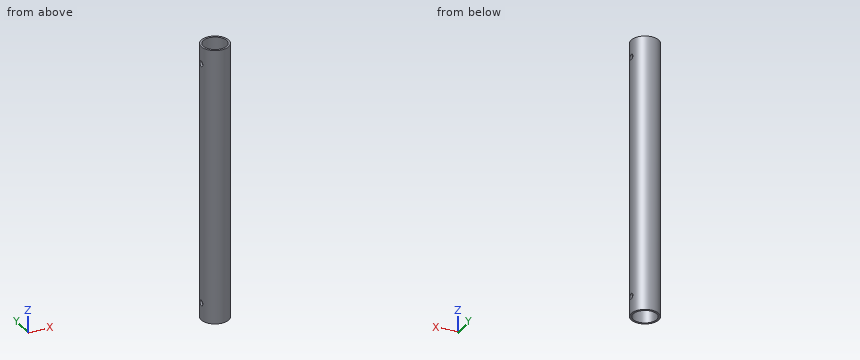
from build123d import *

# Parameters (mm, degrees)
SKETCH1_R           = 10
SKETCH1_R_2         = 8.5
BOSS_EXTRUDE1_DEPTH = 100
SKETCH2_R           = 2
CUT_EXTRUDE1_DEPTH  = 101.995049384


with BuildPart() as part:
    # Sketch1 → Boss-Extrude1 (new body)
    with BuildSketch(Plane.XY):
        Circle(SKETCH1_R)
        Circle(SKETCH1_R_2, mode=Mode.SUBTRACT)
    boss_extrude1 = extrude(amount=BOSS_EXTRUDE1_DEPTH)

    # Sketch2 → Cut-Extrude1 (cut, symmetric)
    with BuildSketch(Plane(origin=(0, 0, 0), x_dir=(0, 0, -1), z_dir=(1, 0, 0))):
        with Locations((-12.5, 0)):
            Circle(SKETCH2_R)
    cut_extrude1 = extrude(amount=CUT_EXTRUDE1_DEPTH, both=True, mode=Mode.SUBTRACT)

    # Mirror1: Boss-Extrude1, Cut-Extrude1 across plane
    add(boss_extrude1.mirror(Plane.XY.offset(100)))
    add(cut_extrude1.mirror(Plane.XY.offset(100)), mode=Mode.SUBTRACT)


solid = part.part
Read the model definition and answer for the solid it produces. Units are mm, in the model's axes. Give positions to 0.01 mm unless a question says otherwise; leave off trailing zeros. Loops run counter-clockwise (first coordinate to the right, second up) from the corner with the lowest first, then second, coordinate; pieces in that order, holes last. Notation, with made-up numbers: M -13,-23.75 L -5,-23.75 A17 ccw -5,-13.75 Z; hole C 47,-1.75 d3. An arc over 180 degrees is marked long. Write each question's results on one line, items separated by ' | '.
1. Straight lines are drawn through the part: line 1 (Y direction, x = 0, z = 148); line 2 (X direction, y = -7.5, z = 39). For each, find the intervals that lie inside material, in ascending order. Write a range as [from, to].
Values:
line 1: y = [-10, -8.5], [8.5, 10] | line 2: x = [-6.61, -4], [4, 6.61]
2. Given pin 1 (1.5 mm diameter, centred on x = -6, z = 61, fed in from -Y); pin 2 (3 mm diameter, centred on y = 6.5, z = 83.5, fed in from +X); pin 3 (2 mm diameter, centred on y = -2, z = 139, fed in from +X), each flat-ended and moving along its own axis, determine where each tip first touches the part or whether it passes through.
Values:
pin 1: stops at y = -8.51 | pin 2: stops at x = 8.66 | pin 3: stops at x = 9.95
3. Section D-D on z = 57.5 is taken. Give the vertices of the cut face in (x, y).
Values:
outline: C 0,0 d20; hole C 0,0 d17
4. Section A-A on x = 0 is taken. Give the vertices of the cut face in (y, z).
Values:
outline: M -10,0 L -8.5,0 L -8.5,200 L -10,200 Z; M 8.5,0 L 10,0 L 10,200 L 8.5,200 Z
5. Section C-C on z = 12.5 is taken. Give the vertices of the cut face in (x, y).
Values:
outline: M -9.8,-2 A10 ccw 9.8,-2 L 8.26,-2 A8.5 cw -8.26,-2 Z; M -9.8,2 L -8.26,2 A8.5 cw 8.26,2 L 9.8,2 A10 ccw Z
6. Section B-B on y = 0 is taken. Give the vertices of the cut face in (x, z).
Values:
outline: M -10,0 L -8.5,0 L -8.5,10.5 L -10,10.5 Z; M -10,14.5 L -8.5,14.5 L -8.5,185.5 L -10,185.5 Z; M -10,189.5 L -8.5,189.5 L -8.5,200 L -10,200 Z; M 8.5,0 L 10,0 L 10,10.5 L 8.5,10.5 Z; M 8.5,14.5 L 10,14.5 L 10,185.5 L 8.5,185.5 Z; M 8.5,189.5 L 10,189.5 L 10,200 L 8.5,200 Z
